```python
from build123d import *

# Parameters (mm, degrees)
PAD_DEPTH = 120


with BuildPart() as part:
    # Sketch → Pad (new body)
    with BuildSketch(Plane.XZ):
        with BuildLine():
            Line((63, 34), (63, -2))
            ThreePointArc((62, -3), (62.707107, -2.707107), (63, -2))
            Line((-23, -3), (62, -3))
            ThreePointArc((-24, -2), (-23.707107, -2.707107), (-23, -3))
            Line((-24, 8), (-24, -2))
            ThreePointArc((-23, 9), (-23.707107, 8.707107), (-24, 8))
            Line((-20, 9), (-23, 9))
            Line((-20, 1), (-20, 9))
            ThreePointArc((-20, 1), (-19.707107, 0.292893), (-19, 0))
            Line((-19, 0), (-5, 0))
            Line((62.110864, 34.542357), (-5, 0))
            ThreePointArc((63, 34), (62.707665, 34.520748), (62.110864, 34.542357))
        make_face()
        with BuildLine():
            Line((2, 0), (59, 0))
            ThreePointArc((59, 0), (59.707107, 0.292893), (60, 1))
            Line((60, 1), (60, 28.381966))
            ThreePointArc((60, 28.381966), (59.525731, 29.232617), (58.552786, 29.276393))
            Line((58.552786, 29.276393), (1.788854, 0.894427))
            ThreePointArc((1.788854, 0.894427), (1.540494, 0.363661), (2, 0))
        make_face(mode=Mode.SUBTRACT)
    extrude(amount=PAD_DEPTH)


solid = part.part
```
For this review, take the finished solid that the model builds, in its own axes (mm). A direction names the side the tool comes from. Coordinates: 2 decimals unless noted, no trailing zeros. Order: outer loops, then holes, each group sorted by start corner. A loop starts at its lowest first (then second) coordinate and runs counter-clockwise, first axis right, second up. Notation, with made-up numbers: (8, -38.5) -> (58, -38.5) arc R18 ccw to (58, -32.5) -> close; hole circle Ø9 at (46, 15). An arc over 180 degrees is marked (long way). Use CSV: the item, a comma, the result in double quotes. Start each with the question number.
Item 1: We need section C-C, the plane x = 39. Give the boundary of the cut face in (y, z), then the cut area to 3 significant figures.
Item 2: We need section B-B, the plane z = 24.5. Give the boundary of the cut face in (x, y), then the cut area to 3 significant figures.
Item 3: For faces 1 (the face through (-12, -59, 0)), 2 (the face through (-21, -59, 9)), 3 (the face through (30.6, -59.2, 15.3)), list the 3-axis set-ups (+Z, -Z, +X, -X, +Y, -Y) from which the entire face can be reached by the end or side of a thin tool; tool diameter is ignored.
Item 4: Wall thickness on probe 1 along X at (y, z) = (-28.5, 6); probe 2 along X at (y, z) = (-96, 20); probe 3 along Z at (x, y) = (-15, -15): over which ranges is each line inside the solid? List them lowest first.
Item 5: We need section A-A, the plane y = -18. Give the boundary of the cut face in (x, z).
Item 6: We need section D-D, the plane z = 3. Give the boundary of the cut face in (x, y), then the cut area to 3 significant figures.
Item 7: Insertion check: pin 1 (17 mm diameter, centred on x = 29, y = -48.5, fed in from +Z) (3 decimals); pin 2 (12 mm diameter, centred on x = 44.5, z = 13.5, fed in from -Y); pin 3 (1 mm diameter, centred on y = -74.5, z = 24, fed in from -X); pin 4 (4 mm diameter, centred on y = -40.5, z = 11.5, fed in from -X). Each pin has a flat end and moves straight along its axis. Give the tip position at first contact, or say it passes through.
Item 8: Draft analysis for pull direction X (two halves, no side actions). For faces 4 (the face through (-20, -59, 5)), 5 (the face through (63, -59, 16)), 6 (the face through (19, -59, -3)), state which applies: pulls with the +X half, pulls with the -X half, needs draft (parallel to the pull), parting line crosses it, or undercut.
Derived:
1,outline,"(-120, -3) -> (0, -3) -> (0, 0) -> (-120, 0) -> close; (-120, 19.5) -> (0, 19.5) -> (0, 22.65) -> (-120, 22.65) -> close"
1,area,"738 mm^2"
2,outline,"(42.6, -120) -> (49, -120) -> (49, 0) -> (42.6, 0) -> close; (60, -120) -> (63, -120) -> (63, 0) -> (60, 0) -> close"
2,area,"1,130 mm^2"
3,face 1,"+Z, +Y, -Y"
3,face 2,"+Z, -X, +Y, -Y"
3,face 3,"+Y, -Y"
4,probe 1,"x = -24 to -20, 6.66 to 12, 60 to 63"
4,probe 2,"x = 33.86 to 40, 60 to 63"
4,probe 3,"z = -3 to 0"
5,outline,"(-24, -2) arc R1 ccw to (-23, -3) -> (62, -3) arc R1 ccw to (63, -2) -> (63, 34) arc R0.61 ccw to (62.11, 34.54) -> (-5, 0) -> (-19, 0) arc R1 cw to (-20, 1) -> (-20, 9) -> (-23, 9) arc R1 ccw to (-24, 8) -> close; hole (1.79, 0.89) arc R0.47 ccw to (2, 0) -> (59, 0) arc R1 ccw to (60, 1) -> (60, 28.38) arc R1 ccw to (58.55, 29.28) -> close"
6,outline,"(-24, -120) -> (-20, -120) -> (-20, 0) -> (-24, 0) -> close; (0.83, -120) -> (6, -120) -> (6, 0) -> (0.83, 0) -> close; (60, -120) -> (63, -120) -> (63, 0) -> (60, 0) -> close"
6,area,"1,460 mm^2"
7,pin 1,"stops at z = 21.875"
7,pin 2,"passes through"
7,pin 3,"stops at x = 40.66"
7,pin 4,"stops at x = 13.46"
8,face 4,"undercut"
8,face 5,"pulls with the +X half"
8,face 6,"needs draft"
